Read the model definition and answer for the solid it produces. Units are mm, in the model's axes. A direction names the side the tool comes from. Coordinates: 2 decimals unless noted, no trailing zeros. Loops run counter-clockwise (first coordinate to the right, second up) from the corner with the lowest first, then second, coordinate; pieces in that order, holes last. Notation, with made-up numbers: (-3.5, 39) -> (12.5, 39) arc R31 cw to (12.5, 63) -> close; hole circle Ø1 at (82, -13.5). An arc over 180 degrees is marked (long way). Answer as CSV lines item,"result".
```python
from build123d import *

# Parameters (mm, degrees)
SKETCH_W        = 100
SKETCH_H        = 100
PAD_DEPTH       = 8
SKETCH001_R     = 2.25
SKETCH001_R_2   = 2.7
SKETCH001_R_3   = 2.6
SKETCH001_R_4   = 2.1
POCKET_DEPTH    = 8.001
SKETCH002_R     = 1.7
POCKET001_DEPTH = 8.001
SKETCH003_R     = 4.6
POCKET002_DEPTH = 5.3
FILLET_R        = 5


with BuildPart() as part:
    # Sketch → Pad (new body)
    with BuildSketch(Plane.XY):
        Rectangle(SKETCH_W, SKETCH_H)
    extrude(amount=PAD_DEPTH)

    # Sketch001 → Pocket (cut, through all)
    with BuildSketch(Plane.XY.offset(8)):
        with Locations((-21, 45)):
            Circle(SKETCH001_R)
        with Locations((-45, 27)):
            Circle(SKETCH001_R)
        with Locations((-45, 45)):
            Circle(SKETCH001_R)
        with Locations((-21, 27)):
            Circle(SKETCH001_R)
        with Locations((21, 27)):
            Circle(SKETCH001_R)
        with Locations((21, 45)):
            Circle(SKETCH001_R)
        with Locations((45, 27)):
            Circle(SKETCH001_R)
        with Locations((45, 45)):
            Circle(SKETCH001_R)
        with Locations((21, -27)):
            Circle(SKETCH001_R)
        with Locations((45, -27)):
            Circle(SKETCH001_R)
        with Locations((45, -45)):
            Circle(SKETCH001_R)
        with Locations((21, -45)):
            Circle(SKETCH001_R)
        with Locations((-21, -27)):
            Circle(SKETCH001_R)
        with Locations((-45, -27)):
            Circle(SKETCH001_R)
        with Locations((-21, -45)):
            Circle(SKETCH001_R)
        with Locations((-45, -45)):
            Circle(SKETCH001_R)
        with Locations((-33, 45)):
            Circle(SKETCH001_R_2)
        with Locations((-33, 25)):
            Circle(SKETCH001_R_2)
        with Locations((33, 45)):
            Circle(SKETCH001_R_3)
        with Locations((33, 25)):
            Circle(SKETCH001_R_3)
        with Locations((-21, -36)):
            Circle(SKETCH001_R_3)
        with Locations((21, -36)):
            Circle(SKETCH001_R_3)
        with Locations((-21, 36)):
            Circle(SKETCH001_R_2)
        with Locations((21, 36)):
            Circle(SKETCH001_R_2)
        with Locations((33, -45)):
            Circle(SKETCH001_R_2)
        with Locations((33, -25)):
            Circle(SKETCH001_R_2)
        with Locations((-33, -25)):
            Circle(SKETCH001_R_2)
        with Locations((-33, -45)):
            Circle(SKETCH001_R_2)
        with Locations((0, 10)):
            Circle(SKETCH001_R_4)
        with Locations((0, 20)):
            Circle(SKETCH001_R_4)
        with Locations((0, 30)):
            Circle(SKETCH001_R_4)
        with Locations((0, 40)):
            Circle(SKETCH001_R_4)
        with Locations((10, 0)):
            Circle(SKETCH001_R_4)
        with Locations((20, 0)):
            Circle(SKETCH001_R_4)
        with Locations((30, 0)):
            Circle(SKETCH001_R_4)
        with Locations((40, 0)):
            Circle(SKETCH001_R_4)
        with Locations((-10, 0)):
            Circle(SKETCH001_R_4)
        with Locations((-20, 0)):
            Circle(SKETCH001_R_4)
        with Locations((-30, 0)):
            Circle(SKETCH001_R_4)
        with Locations((-40, 0)):
            Circle(SKETCH001_R_4)
        with Locations((0, -10)):
            Circle(SKETCH001_R_4)
        with Locations((0, -20)):
            Circle(SKETCH001_R_4)
        with Locations((0, -30)):
            Circle(SKETCH001_R_4)
        with Locations((0, -40)):
            Circle(SKETCH001_R_4)
        Circle(SKETCH001_R_4)
    extrude(amount=-POCKET_DEPTH, mode=Mode.SUBTRACT)

    # Sketch002 → Pocket001 (cut, through all)
    with BuildSketch(Plane.XY.offset(8)):
        with Locations((-10, 10)):
            Circle(SKETCH002_R)
        with Locations((-20, 10)):
            Circle(SKETCH002_R)
        with Locations((-30, 10)):
            Circle(SKETCH002_R)
        with Locations((-40, 10)):
            Circle(SKETCH002_R)
        with Locations((-10, -10)):
            Circle(SKETCH002_R)
        with Locations((-20, -10)):
            Circle(SKETCH002_R)
        with Locations((-30, -10)):
            Circle(SKETCH002_R)
        with Locations((-40, -10)):
            Circle(SKETCH002_R)
        with Locations((10, 10)):
            Circle(SKETCH002_R)
        with Locations((10, -10)):
            Circle(SKETCH002_R)
        with Locations((20, -10)):
            Circle(SKETCH002_R)
        with Locations((20, 10)):
            Circle(SKETCH002_R)
        with Locations((30, 10)):
            Circle(SKETCH002_R)
        with Locations((40, 10)):
            Circle(SKETCH002_R)
        with Locations((30, -10)):
            Circle(SKETCH002_R)
        with Locations((40, -10)):
            Circle(SKETCH002_R)
        with Locations((-10, 20)):
            Circle(SKETCH002_R)
        with Locations((-20, 20)):
            Circle(SKETCH002_R)
        with Locations((10, 20)):
            Circle(SKETCH002_R)
        with Locations((20, 20)):
            Circle(SKETCH002_R)
        with Locations((20, -20)):
            Circle(SKETCH002_R)
        with Locations((10, -20)):
            Circle(SKETCH002_R)
        with Locations((-10, -20)):
            Circle(SKETCH002_R)
        with Locations((-20, -20)):
            Circle(SKETCH002_R)
        with Locations((-10, 30)):
            Circle(SKETCH002_R)
        with Locations((-10, 40)):
            Circle(SKETCH002_R)
        with Locations((10, 40)):
            Circle(SKETCH002_R)
        with Locations((10, 30)):
            Circle(SKETCH002_R)
        with Locations((10, -30)):
            Circle(SKETCH002_R)
        with Locations((-10, -30)):
            Circle(SKETCH002_R)
        with Locations((-10, -40)):
            Circle(SKETCH002_R)
        with Locations((10, -40)):
            Circle(SKETCH002_R)
    extrude(amount=-POCKET001_DEPTH, mode=Mode.SUBTRACT)

    # Sketch003 → Pocket002 (cut)
    with BuildSketch(Plane(origin=(0, 0, 0), x_dir=(1, 0, 0), z_dir=(0, 0, -1))):
        with Locations((-33, 45)):
            Circle(SKETCH003_R)
        with Locations((33, -25)):
            Circle(SKETCH003_R)
        with Locations((33, 25)):
            Circle(SKETCH003_R)
        with Locations((33, 45)):
            Circle(SKETCH003_R)
        with Locations((-33, 25)):
            Circle(SKETCH003_R)
        with Locations((33.027935, -45.104759)):
            Circle(SKETCH003_R)
        with Locations((-32.9375, -44.962784)):
            Circle(SKETCH003_R)
        with Locations((-32.9375, -25.122341)):
            Circle(SKETCH003_R)
    extrude(amount=-POCKET002_DEPTH, mode=Mode.SUBTRACT)

    # Fillet
    fillet_edges = [part.edges().sort_by_distance(p)[0] for p in [
        (-50, -50, 4),
        (50, -50, 4),
        (-50, 50, 4),
        (50, 50, 4),
    ]]
    fillet(fillet_edges, radius=FILLET_R)


solid = part.part
```
Q1. For a pull along Y with two mould halves and no side action, classify faces 1 (the face through (35.47, -28.88, 2.61)), 2 (the face through (-33.351, 27.677, 6.669)) as pulls with the +Y half, pulls with the -Y half, needs draft (parallel to the pull), parting line crosses it, or undercut.
Results:
face 1,"undercut"
face 2,"undercut"
Q2. Find the intervals of material crossed by probe 1 along Y at (x, z) = (45, 3.5); probe 2 along Y at (x, z) = (33, 6.9); probe 3 along X at (y, z) = (-31.5, 3.5), in increasing order. Write a range as [from, to].
Results:
probe 1,"y = [-50, -47.25], [-42.75, -29.25], [-24.75, 24.75], [29.25, 42.75], [47.25, 50]"
probe 2,"y = [-50, -47.7], [-42.3, -27.7], [-22.3, 22.4], [27.6, 42.4], [47.6, 50]"
probe 3,"x = [-50, -10.8], [-9.2, -1.47], [1.47, 9.2], [10.8, 50]"
Q3. For faces 3 (the face through (-30.877, -40.919, 2.613)), 4 (the face through (22.21, 46.897, 4.056)), determine the directions among +Z, -Z, +X, -X, +Y, -Y from which every point of the face is accessible in a straight line to the end or side of a thin tool.
Results:
face 3,"-Z"
face 4,"+Z, -Z"
Q4. A cutting plane is placed at A-A, the plane x = -40. Write down the section's boundary in (y, z).
Results:
outline,"(-50, 0) -> (-11.7, 0) -> (-11.7, 8) -> (-50, 8) -> close; (-8.3, 0) -> (-2.1, 0) -> (-2.1, 8) -> (-8.3, 8) -> close; (2.1, 0) -> (8.3, 0) -> (8.3, 8) -> (2.1, 8) -> close; (11.7, 0) -> (50, 0) -> (50, 8) -> (11.7, 8) -> close"
Q5. A cutting plane is placed at B-B, the plane y = -10. Give the number of separate pieces and of enclosed holes in the cut face, and give its area (3 significant figures).
Results:
separate pieces,"10"
enclosed holes,"0"
area,"549 mm²"
Q6. Given pin 1 Ø5.5 at (x, y) = (30, -10) entering from +Z; pin 2 Ø3 at (x, y) = (33, 43.5) entering from -Z, each flat-ended and moving along its own axis, determine where each tip first touches the part or whether it passes through.
Results:
pin 1,"stops at z = 8"
pin 2,"stops at z = 5.3"
